Can you work these out from the drawing? Everything is in mm from the part's minimum corner. Give positions to 0.01 mm unless a question says otherwise; leave off trailing zeros. Order: outer loops, then holes, each group sorted by start corner. A loop starts at its lowest first (then second) coordinate and runs counter-clockwise, first axis right, second up. Notation, with made-up numbers: M -4.75,19.25 L 49.25,19.25 A10 cw 49.25,32.25 Z; hole C 1,56.25 d6. An arc over 180 degrees is marked long. Use a Markdown table: item, result. Add a question column.
Item 1: Suppose I cut it at B-B on x = 26.25. Write out the boundary of the cut face in (y, z), plus the area to 3 significant figures.
Item 2: If we mould it in two halves opening along Y, with no side actions, what happens to the marked faces 1, 2 and 3? For each: released by +Y, released by -Y, zero draft, split by the parting line, or undercut.
Item 3: If I drill on L1, parallel to Y at x = 26.25, z = 8.75; L2, parallel to X at y = 11.5, z = 9.5 (1 decimal); L3, parallel to Y at x = 9, z = 8.25, over which ranges is the centre line in solid material (lowest first)? Write a range as from..to.
Item 4: Suppose I cut it at A-A on y = 26.25. Write out the boundary of the cut face in (x, z), plus the area to 3 significant figures.
Item 5: I'm going to push flat-ended pins straight in: pin 1 Ø1.2 at (x, y) = (29, 60.5) entering from +Z; pin 2 Ø3 at (y, z) = (10.5, 5.5) entering from +X; pin 3 Ø3 at (y, z) = (31, 8) entering from +X. Where does each tip first touch, or does it pass through?
Item 6: Suppose I cut it at D-D on x = 35.5. Write out the boundary of the cut face in (y, z).
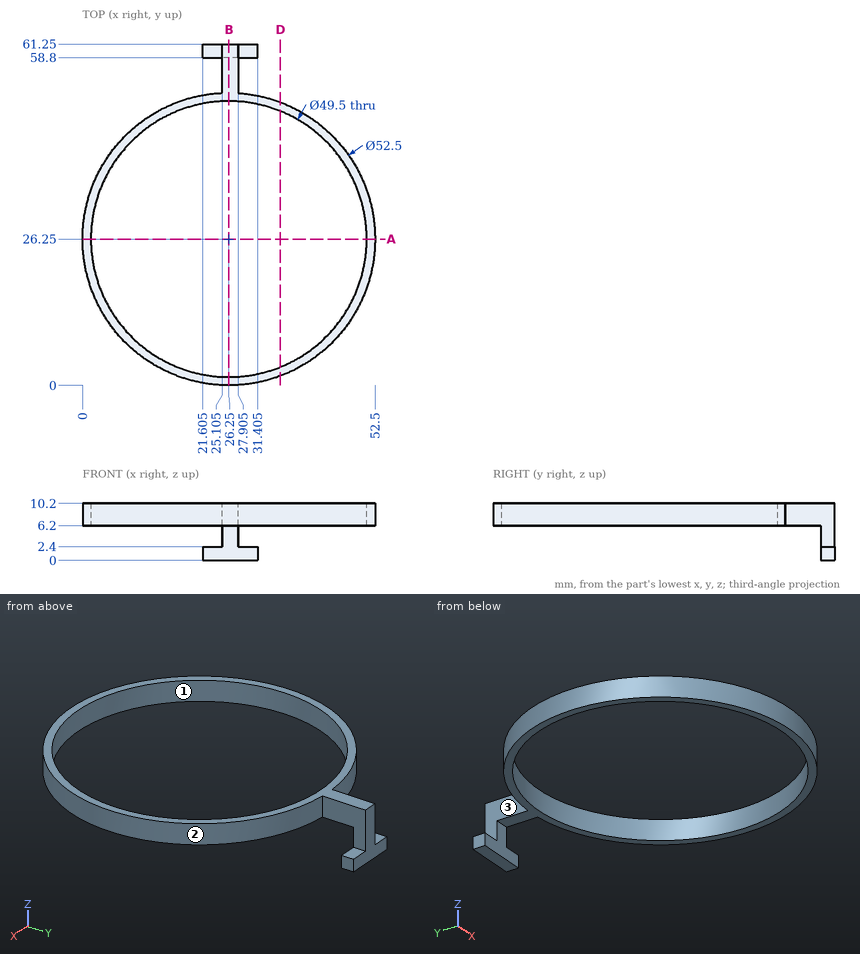
Findings below:
| question | item | result |
|---|---|---|
| 1 | outline | M 0,6.2 L 1.5,6.2 L 1.5,10.2 L 0,10.2 Z; M 51,6.2 L 58.8,6.2 L 58.8,0 L 61.25,0 L 61.25,10.2 L 51,10.2 Z |
| 1 | area | 62.2 mm^2 |
| 2 | face 1 | undercut |
| 2 | face 2 | split by the parting line |
| 2 | face 3 | zero draft |
| 3 | L1 | y = 0..1.5, 51..61.25 |
| 3 | L2 | x = 4.5..6.4, 46.1..48 |
| 3 | L3 | y = 6.46..8.5, 44..46.04 |
| 4 | outline | M 0,6.2 L 1.5,6.2 L 1.5,10.2 L 0,10.2 Z; M 51,6.2 L 52.5,6.2 L 52.5,10.2 L 51,10.2 Z |
| 4 | area | 12.0 mm^2 |
| 5 | pin 1 | stops at z = 2.4 |
| 5 | pin 2 | stops at x = 48.18 |
| 5 | pin 3 | stops at x = 52.3 |
| 6 | outline | M 1.68,6.2 L 3.29,6.2 L 3.29,10.2 L 1.68,10.2 Z; M 49.21,6.2 L 50.82,6.2 L 50.82,10.2 L 49.21,10.2 Z |
